Check sheet for the modelled part. Datum: model origin and axes. Units: mm. A direction names the side the tool comes from. Round coordinates to 2 decimals unless told otherwise and drop trailing zeros. Order: outer loops, then holes, each group sorted by start corner. A loop starts at its lowest first (then second) coordinate and runs counter-clockwise, first axis right, second up. Notation, with made-up numbers: M 36,88 L 93,88 A16 ccw 93,116 Z; hole C 79,31.25 d9. An arc over 180 degrees is marked long. One line per item, written item: value. Start each with the question number.
(1) Cross-section at B-B, the plane z = -41.5. Enter the section's corners in (x, y), and give its area (3 significant figures).
(2) Access from +Z, -Z, +X, -X, +Y, -Y to the whole of each face (thin tool, end or side, straight path). Record for faces 5 (the face through (21.778, 1.479, 80.279)), 6 (the face through (-86.6, 1.5, 30)), 7 (the face through (-8, 0, 2)), 8 (the face through (-80.413, 1.479, -21.279)), 9 (the face through (-11.932, 1.479, 40.666)).
(3) Thickness scan on L1, parallel to X at y = 2.7, z = -18; L2, parallel to X at y = 0.55, z = 27.5; L3, parallel to Z at x = 13, y = 0.2. Record the ranges inside material, lowest first.
(4) Cross-section at C-C, the plane y = 0.5. Count the separate pieces of the cut face and the enclosed holes in it, and give its area (3 significant figures).
(5) Depth check by flat-ended pin: pin 1 Ø1.5 at (x, y) = (15.5, 1) entering from -Z; pin 2 Ø1.5 at (y, z) = (1, 27) entering from -X; pin 3 Ø1.5 at (x, y) = (58.5, 2) entering from -Z. Enter the tip coordinate at first touch or a pass-through.
(6) Release check for a two-part mould opening along Z. For faces 1 (the face through (66.718, 1.479, -115.706)), 2 (the face through (-8, 3, 2)), 3 (the face through (-17.02, 1.48, -29.76)), 4 (the face through (66.85, 1.48, 115.63)) record: released by +Z, released by -Z, zero draft, split by the parting line, or undercut.
(7) Cross-section at D-D, the plane x = -66. Enter the section's corners in (y, z), and give its area (3 significant figures).
(8) Cross-section at A-A, the plane x = -11. Enter the section's corners in (y, z), and give its area (3 significant figures).
Autodesk Inventor part; units mm, degrees
ref_plane "YZ Plane" through (0, 0, 0) normal (1, 0, 0) x (0, 1, 0)
ref_plane "XZ Plane" through (0, 0, 0) normal (0, 1, 0) x (-1, 0, 0)
ref_plane "XY Plane" through (0, 0, 0) normal (0, 0, 1) x (1, 0, 0)
sketch "Sketch1" plane through (0, 0, 0) normal (0, 1, 0) x (-1, 0, 0)
  line L0 (-61.782, 115.6699) -> (131.0641, 4.3301)
  line L1 (131.0641, -4.3301) -> (-61.782, -115.6699)
  line L2 (-69.282, -111.3397) -> (-69.282, 111.3397)
  arc A0 (131.0641, -4.3301) -> (131.0641, 4.3301) centre (128.5641, 0) ccw
  arc A1 (-69.282, -111.3397) -> (-61.782, -115.6699) centre (-64.282, -111.3397) ccw
  arc A2 (-61.782, 115.6699) -> (-69.282, 111.3397) centre (-64.282, 111.3397) ccw
  line L3 (34.641, -60) -> (-45.6615, 79.088)
  line L4 (-69.282, 0) -> (190.0751, 0)
  line L5 (34.641, 60) -> (-41.8401, -72.4692)
  circle A3 centre (0, 0) radius 2.5
  point P0 (0, 0)
  point P1 (-69.282, 120)
  point P2 (-69.282, -120)
  dimension "d5" = 240
  dimension "d9" = 60
  dimension "d10" = 60
  dimension "d14" = 5
  dimension "d25" = 5
extrude "Extrusion1" add sketch "Sketch1" along normal blind 3
sketch "Sketch2" plane through (0, 3, 0) normal (0, 1, 0) x (1, 0, 0)
  point P0 (0, 0)
ref_plane "Work Plane1" through (0, 1.5, 0) normal (0, 1, 0) x (1, 0, 0)
ref_plane "Work Plane2" through (0, 3, 0) normal (0.8660254, 0, 0.5) x (0, 1, 0)
ref_plane "Work Plane3" through (0, 3, 0) normal (-0.8660254, 0, 0.5) x (0, -1, 0)
ref_plane "Work Plane4" through (0, 3, 0) normal (0, 0, 1) x (1, 0, 0)
sketch "Sketch4" plane through (0, 3, 0) normal (0, 1, 0) x (1, 0, 0)
  point P0 (0, 0)
ref_plane "Work Plane5" through (0, 1.5, 0) normal (0, 1, 0) x (1, 0, 0)
ref_plane "Work Plane6" through (51.6025, 3, -19) normal (0, 0, 1) x (1, 0, 0)
sketch "Sketch7" plane through (0, 1.5, 0) normal (0, 1, 0) x (1, 0, 0)
  line L0 (-16.8875, -70.25) -> (-16.8875, -70.25)
  line L1 (-16.8875, -70.25) -> (-16.8875, -70.25)
  line L2 (-25.9808, -65) -> (-18.1865, -69.5)
  line L3 (-14.8875, -66.7859) -> (-16.8875, -70.25)
  line L4 (-14.1375, -65.4869) -> (-19.6375, -75.0131)
  line L5 (-19.6375, -75.0131) -> (-37.824, -64.5131)
  line L6 (-32.324, -54.9869) -> (-19.6375, -75.0131) construction
  line L7 (-37.824, -64.5131) -> (-32.324, -54.9869)
  line L8 (-37.824, -64.5131) -> (-14.1375, -65.4869) construction
  line L9 (-32.324, -54.9869) -> (-14.1375, -65.4869)
  line L10 (-8.4808, -34.6891) -> (-43.4808, -95.3109)
  line L11 (-60.8013, -85.3109) -> (-8.4808, -34.6891) construction
  line L12 (-60.8013, -85.3109) -> (-25.8013, -24.6891)
  line L13 (-25.8013, -24.6891) -> (-43.4808, -95.3109) construction
  line L14 (-7.6865, -51.3135) -> (-15.4808, -46.8135)
  line L15 (-25.9808, -65) -> (-8.4808, -34.6891)
  line L16 (-25.8013, -24.6891) -> (-8.4808, -34.6891)
  line L17 (-16.8875, -70.25) -> (-14.8875, -66.7859)
  line L18 (-18.1865, -69.5) -> (-7.6865, -51.3135)
  line L19 (16.4545, -89.5) -> (-18.1865, -69.5)
  line L20 (-7.6865, -51.3135) -> (26.9545, -71.3135)
  line L21 (26.9545, -71.3135) -> (16.4545, -89.5)
  line L22 (-14.8875, -66.7859) -> (-14.8875, -66.7859)
  line L23 (-43.4808, -95.3109) -> (-60.8013, -85.3109)
  line L24 (-34.641, -60) -> (-25.9808, -65)
  line L25 (-131.0641, -4.3301) -> (61.782, -115.6699)
  line L26 (69.282, 20.5) -> (69.282, 20.5)
  line L27 (69.282, 20.5) -> (69.282, 20.5)
  line L28 (104.282, 10) -> (104.282, -10)
  line L29 (74.782, -0.5) -> (63.782, -0.5)
  line L30 (69.282, 0) -> (69.282, 10)
  line L31 (104.282, -10) -> (34.282, -10)
  line L32 (63.782, -0.5) -> (74.782, 20.5) construction
  line L33 (74.782, 20.5) -> (74.782, -0.5)
  line L34 (104.282, -10) -> (34.282, 10) construction
  line L35 (34.282, -10) -> (104.282, 10) construction
  line L36 (63.782, -0.5) -> (63.782, 20.5)
  line L37 (74.782, -0.5) -> (63.782, 20.5) construction
  line L38 (34.282, -10) -> (34.282, 10)
  line L39 (34.282, 10) -> (104.282, 10)
  line L40 (69.282, 10) -> (34.282, 10)
  line L41 (65.282, 20.5) -> (69.282, 20.5)
  line L42 (65.282, 20.5) -> (65.282, 20.5)
  line L43 (69.282, 20.5) -> (65.282, 20.5)
  line L44 (63.782, 20.5) -> (74.782, 20.5)
  line L45 (69.282, 19) -> (48.282, 19)
  line L46 (69.282, 59) -> (69.282, 19)
  line L47 (69.282, 10) -> (69.282, 19)
  line L48 (48.282, 59) -> (69.282, 59)
  line L49 (48.282, 19) -> (48.282, 10)
  line L50 (48.282, 19) -> (48.282, 59)
  line L51 (-52.3945, 49.75) -> (-52.3945, 49.75)
  line L52 (-52.3945, 49.75) -> (-52.3945, 49.75)
  line L53 (-60.8013, 85.3109) -> (-43.4808, 95.3109)
  line L54 (-36.958, 65.0131) -> (-31.458, 55.4869)
  line L55 (-34.641, 60) -> (-43.3013, 55)
  line L56 (-43.4808, 95.3109) -> (-8.4808, 34.6891)
  line L57 (-31.458, 55.4869) -> (-55.1445, 54.5131) construction
  line L58 (-55.1445, 54.5131) -> (-36.958, 65.0131)
  line L59 (-43.4808, 95.3109) -> (-25.8013, 24.6891) construction
  line L60 (-8.4808, 34.6891) -> (-60.8013, 85.3109) construction
  line L61 (-31.458, 55.4869) -> (-49.6445, 44.9869)
  line L62 (-36.958, 65.0131) -> (-49.6445, 44.9869) construction
  line L63 (-8.4808, 34.6891) -> (-25.8013, 24.6891)
  line L64 (-25.8013, 24.6891) -> (-60.8013, 85.3109)
  line L65 (-43.3013, 55) -> (-25.8013, 24.6891)
  line L66 (-50.3945, 46.2859) -> (-52.3945, 49.75)
  line L67 (-50.3945, 46.2859) -> (-50.3945, 46.2859)
  line L68 (-52.3945, 49.75) -> (-50.3945, 46.2859)
  line L69 (-49.6445, 44.9869) -> (-55.1445, 54.5131)
  line L70 (-51.0955, 50.5) -> (-40.5955, 32.3135)
  line L71 (-85.7365, 30.5) -> (-51.0955, 50.5)
  line L72 (-43.3013, 55) -> (-51.0955, 50.5)
  line L73 (-75.2365, 12.3135) -> (-85.7365, 30.5)
  line L74 (-40.5955, 32.3135) -> (-32.8013, 36.8135)
  line L75 (-40.5955, 32.3135) -> (-75.2365, 12.3135)
  point P0 (0, 0)
  point P1 (-34.641, -60)
  point P2 (-16.8875, -70.25)
  point P3 (-28.7308, -69.7631)
  point P4 (-34.641, -60)
  point P5 (0, 0)
  point P6 (69.282, 111.3397)
  point P7 (69.282, 0)
  point P8 (69.282, 0)
  point P9 (0, 0)
  point P10 (-131.0641, 4.3301)
  point P11 (-34.641, 60)
  point P12 (-34.641, 60)
  point P13 (69.282, 20.5)
  point P14 (74.782, 10)
  point P15 (-52.3945, 49.75)
  point P16 (-46.0513, 59.7631)
  dimension "d59" = 10
  dimension "d60" = 35
  dimension "d61" = 11
  dimension "d62" = 21
  dimension "d63" = 4
  dimension "d64" = 9
  dimension "d65" = 21
  dimension "d66" = 40
  dimension "d129" = 360
extrude "Extrusion3" cut sketch "Sketch7" along normal mid plane 3
ref_plane "Work Plane8" through (-0.6865, 0, 39.1891) normal (-0.8660254, 0, -0.5) x (-0.5, 0, 0.8660254)
sketch "Sketch13" plane through (0, 3, 0) normal (0, 1, 0) x (1, 0, 0)
  circle A0 centre (0, 0) radius 2.75
  dimension "d124" = 5.5
extrude "Extrusion7" cut sketch "Sketch13" against normal through all
ref_plane "Work Plane9" through (-33.5955, 0, -20.1891) normal (0.8660254, 0, -0.5) x (-0.5, 0, -0.8660254)
sketch "Sketch15" plane through (0, 3, 0) normal (0, 1, 0) x (1, 0, 0)
  circle A0 centre (-108.5641, 0) radius 2.5
  circle A1 centre (-108.5641, 0) radius 2.5
  circle A2 centre (54.282, -94.0192) radius 2.5
  circle A3 centre (54.282, 94.0192) radius 2.5
  point P0 (0, 0)
  dimension "d152" = 360
extrude "Extrusion9" cut sketch "Sketch15" against normal blind 10
sketch "Sketch16" plane through (0, 3, 0) normal (0, 1, 0) x (1, 0, 0)
  circle A0 centre (16.6667, -25.1325) radius 2.15
  circle A1 centre (33.9872, -35.1325) radius 2.15
  circle A2 centre (13.432, 27) radius 2.15
  circle A3 centre (13.432, 47) radius 2.15
  circle A4 centre (-47.3442, -11.9974) radius 2.15
  circle A5 centre (-30.0237, -1.9974) radius 2.15
  point P0 (0, 0)
extrude "Extrusion10" cut sketch "Sketch16" against normal through all
sketch "Sketch17" plane through (0, 3, 0) normal (0, 1, 0) x (1, 0, 0)
  line L0 (-25.8013, 24.6891) -> (-8.4808, 34.6891)
  line L1 (-17.141, 29.6891) -> (-7.7719, 13.4613)
  line L2 (-8.4808, 34.6891) -> (-25.8013, 24.6891)
  line L3 (-17.141, 29.6891) -> (-12.141, 21.0289)
  circle A0 centre (-12.141, 21.0289) radius 7.5
  circle A1 centre (-12.141, -21.0289) radius 7.5
  circle A2 centre (24.282, 0) radius 7.5
  point P0 (0, 0)
  dimension "d158" = 10
  dimension "d159" = 15
  dimension "d162" = 360
extrude "Extrusion11" cut sketch "Sketch17" against normal blind 10
properties part number "baseplate" material "PET Plastic"
Values found:
1. outline: M -12.41,0 L 48.28,0 L 48.28,3 L -12.41,3 Z
1. area: 182 mm^2
2. face 5: -X, +Y, -Y
2. face 6: +Z, -X, +Y, -Y
2. face 7: +Z, -Z, +X, -X, -Y
2. face 8: -Z, +Y, -Y
2. face 9: +Y, -Y
3. L1: -107.39 to -78.52, -65.39 to -19, -5.28 to 48.28
3. L2: -90.93 to -27.42, -20.93 to -15.93, -8.35 to 69.28
3. L3: -87.51 to -49.11, -44.89 to -29.11, -24.89 to 63.26
4. separate pieces: 1
4. enclosed holes: 13
4. area: 19,000 mm^2
5. pin 1: z = -89.38
5. pin 2: x = -93.1
5. pin 3: z = -114.21
6. face 1: released by -Z
6. face 2: zero draft
6. face 3: undercut
6. face 4: released by +Z
7. outline: M 0,-17.65 L 3,-17.65 L 3,41.89 L 0,41.89 Z
7. area: 179 mm^2
8. outline: M 0,-73.65 L 3,-73.65 L 3,-39.05 L 0,-39.05 Z; M 0,-33.23 L 3,-33.23 L 3,-28.44 L 0,-28.44 Z; M 0,-13.62 L 3,-13.62 L 3,13.62 L 0,13.62 Z; M 0,28.44 L 3,28.44 L 3,33.23 L 0,33.23 Z; M 0,39.05 L 3,39.05 L 3,49.4 L 0,49.4 Z
8. area: 245 mm^2
